Answer from the drawing. Dimensions are ordinates in mm from the lowest x, y and z of the part. A direction names the side the tool comes from. Coordinates: 2 decimals unless noted, no trailing zeros. Order: outer loops, then holes, each group sorted by start corner. A loop starts at its lowest first (then second) coordinate and runs counter-clockwise, first axis right, second up. Notation, with made-up numbers: (15.25, 9) - (57.25, 9) arc R28 cw to (57.25, 28) - close; hole circle Ø8 at (16.25, 10). An arc over 180 degrees is marked (long way). Use a Markdown table: item, result. Add a question column.
Item 1: The part is cut by section A-A, the plane x = 6. Give the vertices of the cut face in (y, z), then the cut area to 4 significant figures.
Item 2: The part is cut by section D-D, the plane z = 63.5. Give the vertices of the cut face in (x, y).
Item 3: For the marked faces 1 and 2, determine the directions among +Z, -Z, +X, -X, +Y, -Y from which every point of the face is accessible in a straight line to the end or side of a thin tool.
Item 4: The part is cut by section C-C, the plane y = 30.5. Give the vertices of the cut face in (x, z).
Item 5: Flat-ended cylindrical pins translate along their axes: P1, Ø2, axis at x = 14.5, z = 24.5, coming from the +Y side; P2, Ø6, axis at y = 25.5, z = 42.5, coming from the -X side; P3, Ø4, axis at x = 2.5, y = 6, coming from the +Z side. Find the tip coordinate at first contact, or state that the pin passes through.
Item 6: The part is cut by section B-B, the plane z = 9.5. Give the vertices of the cut face in (x, y), then the cut area to 3 significant figures.
Item 7: Find the intervals of material crossed by line 1 along Y through (x, z) = (24, 21.5); line 2 along X through (y, z) = (17, 33), in increasing order.
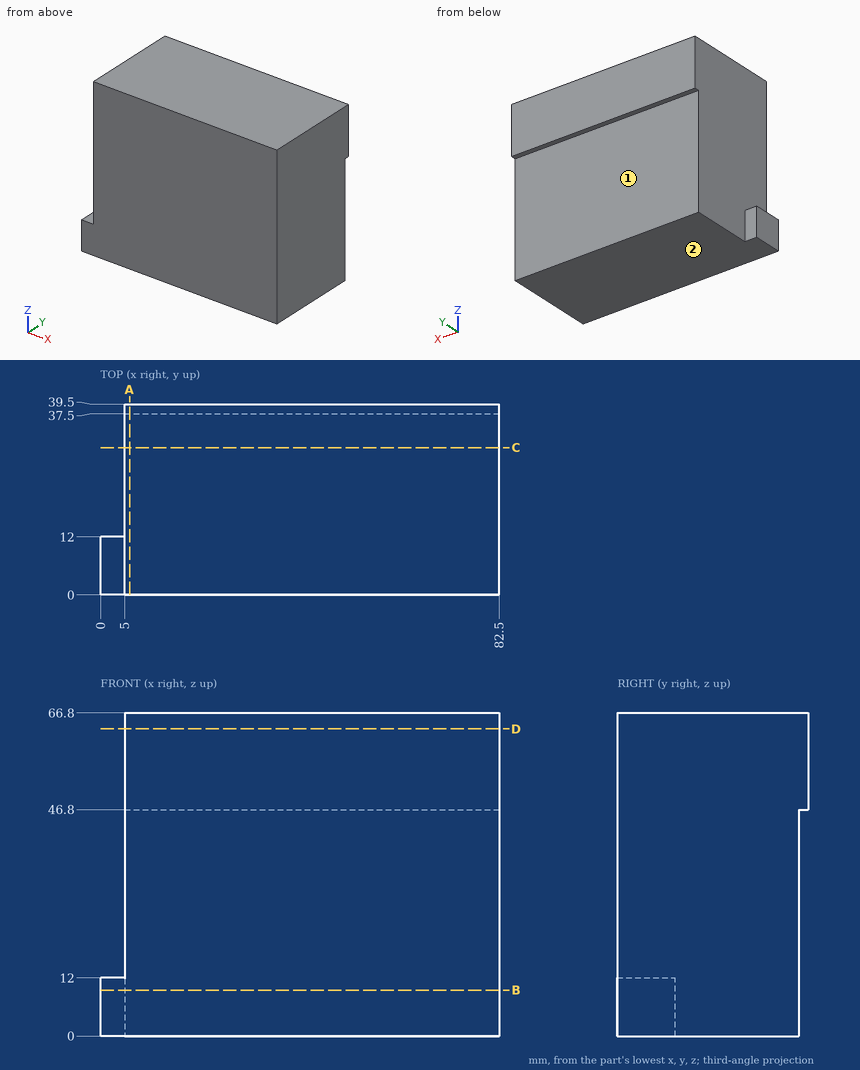
Solution:
| question | item | result |
|---|---|---|
| 1 | outline | (0, 0) - (37.5, 0) - (37.5, 46.8) - (39.5, 46.8) - (39.5, 66.8) - (0, 66.8) - close |
| 1 | area | 2,545 mm2 |
| 2 | outline | (5, 0) - (82.5, 0) - (82.5, 39.5) - (5, 39.5) - close |
| 3 | face 1 | -Z, +X, -X, +Y |
| 3 | face 2 | -Z, +X, -X, +Y, -Y |
| 4 | outline | (5, 0) - (82.5, 0) - (82.5, 66.8) - (5, 66.8) - close |
| 5 | P1 | stops at y = 37.5 |
| 5 | P2 | stops at x = 5 |
| 5 | P3 | stops at z = 12 |
| 6 | outline | (0, 0) - (82.5, 0) - (82.5, 37.5) - (5, 37.5) - (5, 12) - (0, 12) - close |
| 6 | area | 2,970 mm2 |
| 7 | line 1 | y = 0 to 37.5 |
| 7 | line 2 | x = 5 to 82.5 |
